CAD build for the part. Positions are in the model's coordinates, mm. Coordinates: 2 decimals unless noted, no trailing zeros. Write each loop counter-clockwise with the first axis right and the second up, starting at its lowest first coordinate (ties: lowest second). Pieces come first, ordered by that corner, then holes.
```python
from build123d import *

# Parameters (mm, degrees)
SKETCH1_R           = 23
SKETCH1_R_2         = 21.5
BOSS_EXTRUDE1_DEPTH = 40
SKETCH2_W           = 60
SKETCH2_H           = 20
CUT_EXTRUDE1_DEPTH  = 20


with BuildPart() as part:
    # Sketch1 → Boss-Extrude1 (new body)
    with BuildSketch(Plane(origin=(0, 0, 0), x_dir=(1, 0, 0), z_dir=(0, 1, 0))):
        with Locations(Location((0, 0, 0), (0, 0, 270))):
            Circle(SKETCH1_R)
        with Locations(Location((0, 0, 0), (0, 0, 270))):
            Circle(SKETCH1_R_2, mode=Mode.SUBTRACT)
    extrude(amount=BOSS_EXTRUDE1_DEPTH)

    # Sketch2 → Cut-Extrude1 (cut)
    with BuildSketch(Plane(origin=(0, 40, 0), x_dir=(1, 0, 0), z_dir=(0, 1, 0))):
        Rectangle(SKETCH2_W, SKETCH2_H)
    extrude(amount=-CUT_EXTRUDE1_DEPTH, mode=Mode.SUBTRACT)


solid = part.part
```
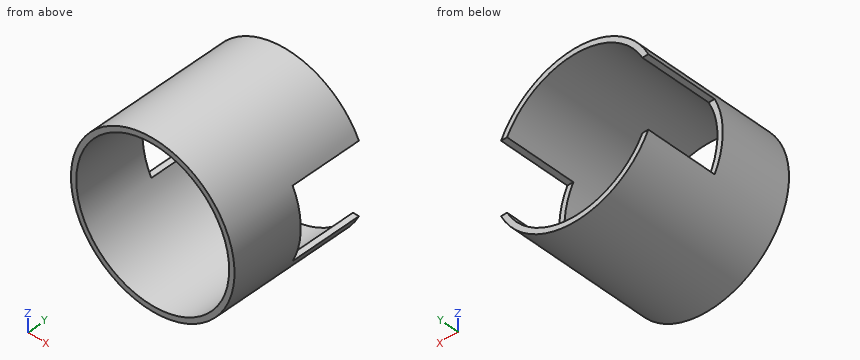
Item 1: Saw through at A-A, the plane x = 10. Write the cut outline in (y, z).
Item 2: Flat gauge pins, fed straight in: pin 1 Ø1.5 at (x, y) = (17.5, 9) entering from +Z; pin 2 Ø1.8 at (x, y) = (-19.5, 29.5) entering from -Z; pin 3 Ø8 at (x, y) = (-7.5, 11.5) entering from -Z. Where does each tip first touch, or does it go through?
Item 3: Saw through at C-C, the plane x = -20. Write the cut outline in (y, z).
Item 4: Saw through at B-B, the plane y = 35. Write the cut outline in (x, z).
Item 5: Saw through at D-D, the plane y = 2.5. Write the cut outline in (x, z), and give its area (3 significant figures).
Item 6: Wall check: line 1 along Z through (x, y) = (0, 21.5); line 2 along Z through (x, y) = (13, 8). Give the ranges that are in metal, low to high.
Working result:
1. outline: (0, -20.71) - (40, -20.71) - (40, -19.03) - (0, -19.03) - close; (0, 19.03) - (40, 19.03) - (40, 20.71) - (0, 20.71) - close
2. pin 1: stops at z = 15.76
2. pin 2: stops at z = -13.53
2. pin 3: stops at z = -22.73
3. outline: (0, -11.36) - (40, -11.36) - (40, -10) - (20, -10) - (20, -7.89) - (0, -7.89) - close; (0, 7.89) - (20, 7.89) - (20, 10) - (40, 10) - (40, 11.36) - (0, 11.36) - close
4. outline: (-20.71, -10) arc R23 ccw to (20.71, -10) - (19.03, -10) arc R21.5 cw to (-19.03, -10) - close; (-20.71, 10) - (-19.03, 10) arc R21.5 cw to (19.03, 10) - (20.71, 10) arc R23 ccw to start
5. outline: circle Ø46 at (0, 0); hole circle Ø43 at (0, 0)
5. area: 210 mm2
6. line 1: z = -23 to -21.5, 21.5 to 23
6. line 2: z = -18.97 to -17.12, 17.12 to 18.97
